Design review of the part built by this model. Coordinates are the model's own, in mm. A direction names the side the tool comes from. Coordinates: 2 decimals unless noted, no trailing zeros. Loops run counter-clockwise (first coordinate to the right, second up) from the corner with the lowest first, then second, coordinate; pieces in that order, holes last.
Autodesk Inventor part; units mm, degrees
ref_plane "YZ Plane" through (0, 0, 0) normal (1, 0, 0) x (0, 1, 0)
ref_plane "XZ Plane" through (0, 0, 0) normal (0, 1, 0) x (-1, 0, 0)
ref_plane "XY Plane" through (0, 0, 0) normal (0, 0, 1) x (1, 0, 0)
sketch "스케치1" plane through (0, 0, 0) normal (0, 1, 0) x (-1, 0, 0)
  circle A0 centre (0, 0) radius 37
  circle A1 centre (0, 0) radius 21 construction
  circle A2 centre (0, -21) radius 1.65
  circle A3 centre (18.1865, 10.5) radius 1.65
  circle A4 centre (-18.1865, 10.5) radius 1.65
  dimension "d1" = 42
  dimension "d0" = 74
  dimension "d2" = 3.3
  dimension "d6" = 360
extrude "돌출1" add sketch "스케치1" along normal blind 3
sketch "스케치2" plane through (0, 0, 0) normal (0, -1, 0) x (1, 0, 0)
  line L0 (60, 50) -> (-60, 50)
  line L1 (-60, 50) -> (-60, -50)
  line L2 (-60, -50) -> (60, -50)
  line L3 (60, -50) -> (60, 50)
  line L4 (60, 50) -> (-60, -50) construction
  line L5 (-60, 50) -> (60, -50) construction
  circle A0 centre (0, 0) radius 37
  circle A1 centre (18.1865, 10.5) radius 1.65
  circle A2 centre (-18.1865, 10.5) radius 1.65
  circle A3 centre (0, -21) radius 1.65
  dimension "d10" = 120
  dimension "d11" = 100
extrude "돌출2" add sketch "스케치2" along normal blind 7.5 contours L3 L2 L1 L0 | A0
fillet "모깎기1" radius 2 4 edges at (60, 0, 0) (0, 0, -50) (-60, 0, 0) (0, 0, 50)
fillet "모깎기1" radius 1 1 edges at (37, 3, 0)
sketch "스케치5" plane through (0, -7.5, 0) normal (0, -1, 0) x (1, 0, 0)
  circle A0 centre (0, 0) radius 36
extrude "돌출3" cut sketch "스케치5" against normal blind 7.5
sketch "스케치6" plane through (0, -7.5, 0) normal (0, -1, 0) x (1, 0, 0)
  circle A0 centre (-50, -40) radius 3.1
  line L0 (-60, -50) -> (60, -50)
  line L1 (-60, 50) -> (-60, -50)
  circle A1 centre (50, -40) radius 3.1
  circle A2 centre (-50, 40) radius 3.1
  circle A3 centre (50, 40) radius 3.1
  point P0 (0, 0)
  dimension "d18" = 6.2
  dimension "d19" = 10
  dimension "d20" = 10
  dimension "d21" = 120
  dimension "d22" = 100
  dimension "d25" = 100
  dimension "d32" = 80
extrude "돌출4" cut sketch "스케치6" against normal through all
sketch "스케치7" plane through (0, 0, 0) normal (0, 1, 0) x (1, 0, 0)
  circle A0 centre (-50, 40) radius 3.1
  circle A1 centre (50, 40) radius 3.1
  circle A2 centre (-50, -40) radius 3.1
  circle A3 centre (50, -40) radius 3.1
  circle A4 centre (0, 0) radius 37
  line L0 (-58, -48) -> (-58, 48)
  line L1 (58, -48) -> (-58, -48)
  line L2 (58, 48) -> (58, -48)
  line L3 (-58, 48) -> (58, 48)
  circle A5 centre (50, -40) radius 5.5
  circle A6 centre (-50, -40) radius 5.5
  circle A7 centre (-50, 40) radius 5.5
  circle A8 centre (50, 40) radius 5.5
  dimension "d39" = 11
  dimension "d40" = 11
  dimension "d41" = 11
  dimension "d42" = 11
extrude "돌출5" cut sketch "스케치7" against normal blind 4 contours A5 | A6 | A7 | A8
properties part number "LiDAR_holder_upper" material "ABS Plastic"
Q1. Take a section at C-C, the plane x = 50. Write out the cut boundary in (y, z).
Q2. Take a section at A-A, the plane x = 0. Write out the cut boundary in (y, z).
Q3. Take a section at B-B, the plane z = 40. Write out the cut boundary in (x, y).
Q4. Machinability: for faces 1 (the flat face through (-47.6, -4, -37.6)), 2 (the flat face through (-1, 0, 1)), 3 (the flat face through (1, 3, 1)), which of the approach directions +Z, -Z, +X, -X, +Y, -Y give a long, thin tool a straight path to every point of the face, cutting with its end or side? Answer none if there is none.
Q5. Take a section at D-D, the plane z = 10.5. Give the number of separate pieces and of enclosed holes in the cut face, then the cut area to 3 significant figures.
Q6. For line 1 (Z direction, x = 50, y = -2.7); line 2 (X direction, y = -6.35, z = -40); line 3 (Z direction, x = -45.5, y = -2.25), list the stretches that pass through material, from the lowest coordinate up.
Q7. Clearance check with flat-ended pins moving along their axes: pin 1 Ø3 at (x, z) = (18.19, 10.5) entering from -Y; pin 2 Ø10 at (x, z) = (50, -40) entering from +Y; pin 3 Ø4 at (x, z) = (0, -21) entering from -Y; pin 4 Ø9 at (x, z) = (48, -40.5) entering from +Y. State where each tip first meets the part, or that it passes through.
Q8. The part is to be moulded in two halves that separate along X. For faces 4 (the cylindrical face through (8.02, 0.99, 36.12)), 5 (the flat face through (1, -5, 50)), 6 (the cylindrical face through (-50.404, -5.774, -36.926)), say which applies: pulls with the +X half, pulls with the -X half, needs draft (parallel to the pull), parting line crosses it, or undercut.
Entries:
1. outline: (-7.5, -50) - (-2, -50) arc R2 ccw to (0, -48) - (0, -45.5) - (-4, -45.5) - (-4, -43.1) - (-7.5, -43.1) - close; (-7.5, -36.9) - (-4, -36.9) - (-4, -34.5) - (0, -34.5) - (0, 34.5) - (-4, 34.5) - (-4, 36.9) - (-7.5, 36.9) - close; (-7.5, 43.1) - (-4, 43.1) - (-4, 45.5) - (0, 45.5) - (0, 48) arc R2 ccw to (-2, 50) - (-7.5, 50) - close
2. outline: (-7.5, -50) - (-2, -50) arc R2 ccw to (0, -48) - (0, -37) - (2, -37) arc R1 ccw to (3, -36) - (3, -22.65) - (0, -22.65) - (0, -36) - (-7.5, -36) - close; (-7.5, 36) - (0, 36) - (0, -19.35) - (3, -19.35) - (3, 36) arc R1 ccw to (2, 37) - (0, 37) - (0, 48) arc R2 ccw to (-2, 50) - (-7.5, 50) - close
3. outline: (-60, -7.5) - (-53.1, -7.5) - (-53.1, -4) - (-55.5, -4) - (-55.5, 0) - (-58, 0) arc R2 ccw to (-60, -2) - close; (-46.9, -7.5) - (46.9, -7.5) - (46.9, -4) - (44.5, -4) - (44.5, 0) - (-44.5, 0) - (-44.5, -4) - (-46.9, -4) - close; (53.1, -7.5) - (60, -7.5) - (60, -2) arc R2 ccw to (58, 0) - (55.5, 0) - (55.5, -4) - (53.1, -4) - close
4. face 1: +Y
4. face 2: -Y
4. face 3: +Z, -Z, +X, -X, +Y
5. separate pieces: 3
5. enclosed holes: 0
5. area: 574 mm2
6. line 1: z = -50 to -45.5, -34.5 to 34.5, 45.5 to 50
6. line 2: x = -60 to -53.1, -46.9 to 46.9, 53.1 to 60
6. line 3: z = -50 to -43.16, -36.84 to 36.84, 43.16 to 50
7. pin 1: passes through
7. pin 2: stops at y = -4
7. pin 3: stops at y = 0
7. pin 4: stops at y = 0
8. face 4: parting line crosses it
8. face 5: needs draft
8. face 6: undercut
